Input: part model. Units: mm. Frame: model coordinates. Face numbers are marked on the shaded views. Round coordinates to 2 decimals unless told otherwise and drop trailing zeros. Loops run counter-clockwise (first coordinate to the right, second up) from the corner with the lowest first, then second, coordinate; pieces in that order, holes last. Notation, with made-up numbers: (17.5, 18) - (50.5, 18) arc R22 cw to (50.5, 54) - close; hole circle Ø9 at (75.25, 62). An arc over 180 degrees is marked (long way). Write each question's results on one line, items separated by ' | '.
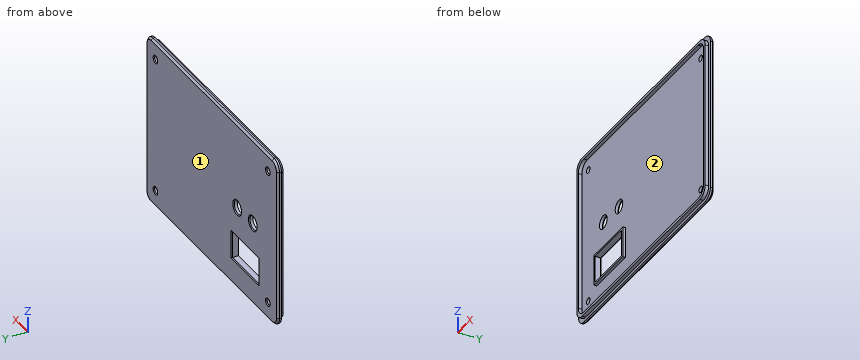
Autodesk Inventor part; units mm, degrees
ref_plane "YZ Plane" through (0, 0, 0) normal (1, 0, 0) x (0, 1, 0)
ref_plane "XZ Plane" through (0, 0, 0) normal (0, 1, 0) x (-1, 0, 0)
ref_plane "XY Plane" through (0, 0, 0) normal (0, 0, 1) x (1, 0, 0)
sketch "Sketch1" plane through (0, 0, 0) normal (0, 1, 0) x (-1, 0, 0)
  line L0 (66.5812, -42.2738) -> (-55.4188, -42.2738)
  line L1 (-55.4188, -42.2738) -> (-55.4188, 46.7262)
  line L2 (-55.4188, 46.7262) -> (66.5812, 46.7262)
  line L3 (66.5812, 46.7262) -> (66.5812, -42.2738)
  point P0 (0, 0)
  dimension "d0" = 122
  dimension "d1" = 89
extrude "Extrusion1" add sketch "Sketch1" along normal blind 2
sketch "Sketch2" plane through (0, 0, 0) normal (0, -1, 0) x (1, 0, 0)
  line L0 (53.8188, -40.6738) -> (-64.9812, -40.6738)
  line L1 (-64.9812, -40.6738) -> (-64.9812, 45.1262)
  line L2 (-64.9812, 45.1262) -> (53.8188, 45.1262)
  line L3 (53.8188, 45.1262) -> (53.8188, -40.6738)
  line L4 (55.4188, -42.2738) -> (-66.5812, -42.2738)
  line L5 (55.4188, 46.7262) -> (55.4188, -42.2738)
  line L6 (-66.5812, 46.7262) -> (55.4188, 46.7262)
  line L7 (-66.5812, -42.2738) -> (-66.5812, 46.7262)
  line L8 (52.4188, -39.2738) -> (-63.5812, -39.2738)
  line L9 (-63.5812, -39.2738) -> (-63.5812, 43.7262)
  line L10 (-63.5812, 43.7262) -> (52.4188, 43.7262)
  line L11 (52.4188, 43.7262) -> (52.4188, -39.2738)
  point P0 (0, 0)
  dimension "d4" = 1.6
  dimension "d5" = 1.6
  dimension "d6" = 1.6
  dimension "d7" = 1.6
  dimension "d8" = 1.4
  dimension "d9" = 1.4
  dimension "d10" = 1.4
  dimension "d11" = 1.4
extrude "Extrusion2" add sketch "Sketch2" along normal blind 1.8 contours L0 L1 L2 L3
sketch "Sketch3" plane through (0, 2, 0) normal (0, 1, 0) x (1, 0, 0)
  line L0 (55.4188, 42.2738) -> (-66.5812, 42.2738)
  line L1 (-66.5812, 42.2738) -> (-66.5812, -46.7262)
  point P0 (0, 0)
  point P1 (-57.5812, 33.2738)
  dimension "d14" = 9
  dimension "d15" = 9
hole "Hole1" at (-57.5812, 2, -33.2738) direction (0, -1, 0) diameter 3.2 end through all
pattern_linear "Rectangular Pattern1" count 2 spacing 71 along (0, 0, 1) count 2 spacing 104 along (1, 0, 0) of "Hole1"
fillet "Fillet1" radius 5 12 edges at (-66.5812, 1, 46.7262) (-64.9812, -0.9, 45.1262) (-63.5812, -0.9, 43.7262) (-66.5812, 1, -42.2738) (-64.9812, -0.9, -40.6738) (-63.5812, -0.9, -39.2738) (55.4188, 1, -42.2738) (53.8188, -0.9, -40.6738) (52.4188, -0.9, -39.2738) (52.4188, -0.9, 43.7262) (53.8188, -0.9, 45.1262) (55.4188, 1, 46.7262)
chamfer "Chamfer1" distance 1 angle 45 8 edges at (-5.5812, 2, -42.2738) (-65.1167, 2, -40.8093) (-66.5812, 2, 2.2262) (-65.1167, 2, 45.2618) (-5.5812, 2, 46.7262) (53.9543, 2, 45.2618) (55.4188, 2, 2.2262) (53.9543, 2, -40.8093)
sketch "Sketch4" plane through (0, 2, 0) normal (0, 1, 0) x (1, 0, 0)
  line L0 (-48.8812, 28.5738) -> (-24.1812, 28.5738)
  line L1 (-24.1812, 28.5738) -> (-24.1812, 14.5738)
  line L2 (-24.1812, 14.5738) -> (-48.8812, 14.5738)
  line L3 (-48.8812, 14.5738) -> (-48.8812, 28.5738)
  line L4 (50.4188, 42.2738) -> (-61.5812, 42.2738)
  line L5 (-66.5812, 37.2738) -> (-66.5812, -41.7262)
  circle A0 centre (-43.6812, -1.3962) radius 3.5
  circle A1 centre (-29.1812, -1.3962) radius 3.5
  point P0 (0, 0)
  dimension "d33" = 24.7
  dimension "d34" = 14
  dimension "d35" = 13.7
  dimension "d36" = 17.7
  dimension "d37" = 7
  dimension "d38" = 7
  dimension "d39" = 22.9
  dimension "d40" = 14.5
  dimension "d41" = 43.67
  dimension "d42" = 43.67
extrude "Extrusion3" cut sketch "Sketch4" against normal through all
sketch "Sketch5" plane through (0, 0, 0) normal (0, -1, 0) x (1, 0, 0)
  line L0 (-48.8812, -14.5738) -> (-24.1812, -14.5738)
  line L1 (-48.8812, -14.5738) -> (-24.1812, -14.5738)
  line L2 (-24.1812, -14.5738) -> (-24.1812, -28.5738)
  line L3 (-24.1812, -28.5738) -> (-48.8812, -28.5738)
  line L4 (-48.8812, -28.5738) -> (-48.8812, -14.5738)
  line L5 (-49.8812, -13.5738) -> (-23.1812, -13.5738)
  line L6 (-23.1812, -13.5738) -> (-23.1812, -29.5738)
  line L7 (-23.1812, -29.5738) -> (-49.8812, -29.5738)
  line L8 (-49.8812, -29.5738) -> (-49.8812, -13.5738)
  point P0 (0, 0)
  dimension "d45" = 1
  dimension "d46" = 1
  dimension "d47" = 1
  dimension "d48" = 1
extrude "Extrusion4" add sketch "Sketch5" along normal blind 1.4
chamfer "Chamfer2" distance 0.5 angle 45 10 edges at (-47.1812, 2, 1.3962) (-48.8812, 2, -21.5738) (-36.5312, 2, -14.5738) (-36.5312, 2, -28.5738) (-24.1812, 2, -21.5738) (-32.6812, 2, 1.3962) (46.4188, 2, 36.1262) (-57.5812, 2, 36.1262) (-57.5812, 2, -34.8738) (46.4188, 2, -34.8738)
equation "\"d5\" = d4"
equation "\"d6\" = d4"
equation "\"d7\" = d4"
equation "\"d9\" = d8"
equation "\"d10\" = d8"
equation "\"d11\" = d8"
equation "\"d42\" = d41"
equation "\"d46\" = d45"
equation "\"d47\" = d45"
equation "\"d48\" = d45"
properties part number "housing_top_v_2"
1. Section query C-C, the plane z = 32.5. Output: boundary loops of the cut face in (x, y).
Answer:
outline: (-66.58, 0) - (-64.98, 0) - (-64.98, -1.8) - (-63.58, -1.8) - (-63.58, 0) - (52.42, 0) - (52.42, -1.8) - (53.82, -1.8) - (53.82, 0) - (55.42, 0) - (55.42, 1) - (54.42, 2) - (-65.58, 2) - (-66.58, 1) - close
2. Section query B-B, the plane x = 29. Output: boundary loops of the cut face in (y, z).
Answer:
outline: (-1.8, -40.67) - (0, -40.67) - (0, -42.27) - (1, -42.27) - (2, -41.27) - (2, 45.73) - (1, 46.73) - (0, 46.73) - (0, 45.13) - (-1.8, 45.13) - (-1.8, 43.73) - (0, 43.73) - (0, -39.27) - (-1.8, -39.27) - close
3. Contact query for flat-ended pins moving along their axis: pin 1 (1.9 mm diameter, centred on x = -57.58, z = 37.73, fed in from +Y); pin 2 (10 mm diameter, centred on x = -16.5, z = -3, fed in from -Y); pin 3 (1 mm diameter, centred on y = -1, z = -3.5, fed in from -X); pin 4 (0.5 mm diameter, centred on x = 18, y = -1, fed in from +Z). Output: stop coordinate, or through.
Answer:
pin 1: through | pin 2: y = 0 | pin 3: x = -64.98 | pin 4: z = 45.13
4. Line query: line 1 (X direction, y = -0.4, z = -15); line 2 (X direction, y = -1.5, z = -13.5); line 3 (Z direction, x = 31, y = -0.8). Output: solid intervals per line, ascending. Write a range as [from, to].
Answer:
line 1: [-64.98, -63.58], [-49.88, -48.88], [-24.18, -23.18], [52.42, 53.82] | line 2: [-64.98, -63.58], [52.42, 53.82] | line 3: [-40.67, -39.27], [43.73, 45.13]
5. Section query A-A, the plane z = -19.5. Output: boundary loops of the cut face in (x, y).
Answer:
outline: (-66.58, 0) - (-64.98, 0) - (-64.98, -1.8) - (-63.58, -1.8) - (-63.58, 0) - (-49.88, 0) - (-49.88, -1.4) - (-48.88, -1.4) - (-48.88, 1.5) - (-49.38, 2) - (-65.58, 2) - (-66.58, 1) - close; (-24.18, -1.4) - (-23.18, -1.4) - (-23.18, 0) - (52.42, 0) - (52.42, -1.8) - (53.82, -1.8) - (53.82, 0) - (55.42, 0) - (55.42, 1) - (54.42, 2) - (-23.68, 2) - (-24.18, 1.5) - close
6. Mould query, pull axis X, two halves, no side actions, for the marked faces 1 and 2. Classes: pulls with the +X half, pulls with the -X half, needs draft (parallel to the pull), parting line crosses it, or undercut.
Answer:
face 1: needs draft | face 2: undercut
